The model under review builds one solid part; all positions refer to its coordinate system, in mm. Face numbers are marked on the shaded views. A direction names the side the tool comes from. Round coordinates to 2 decimals unless told otherwise and drop trailing zeros. Order: outer loops, then holes, each group sorted by start corner. A loop starts at its lowest first (then second) coordinate and runs counter-clockwise, first axis right, second up.
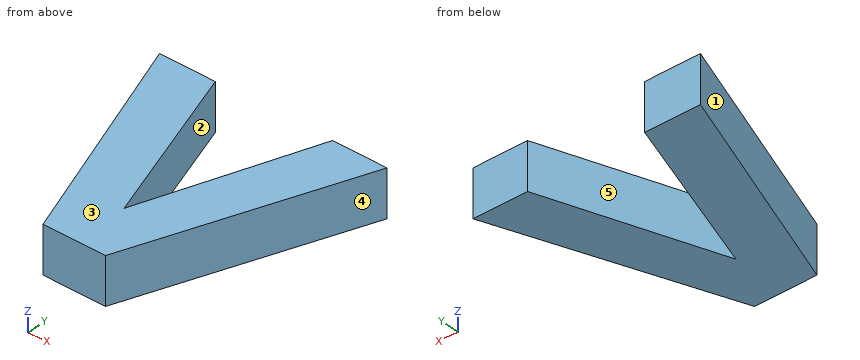
Autodesk Inventor part; units mm, degrees
ref_plane "YZ Plane" through (0, 0, 0) normal (1, 0, 0) x (0, 1, 0)
ref_plane "XZ Plane" through (0, 0, 0) normal (0, 1, 0) x (-1, 0, 0)
ref_plane "XY Plane" through (0, 0, 0) normal (0, 0, 1) x (1, 0, 0)
sketch "Sketch1" plane through (0, 0, 0) normal (0, 0, 1) x (1, 0, 0)
  line L0 (-20, -20) -> (20, -20)
  line L1 (20, -20) -> (20, 20)
  line L2 (20, 20) -> (-20, 20)
  line L3 (-20, 20) -> (-20, -20)
  line L4 (-20, 0) -> (20, 0) construction
  line L5 (0, -28) -> (0, 28) construction
  line L6 (-28, 0) -> (28, 0) construction
  point P0 (0, 0)
  dimension "d0" = 40
extrude "Extrusion1" add sketch "Sketch1" along normal blind 1.4
sketch "Sketch2" plane through (0, 0, 1.4) normal (0, 0, 1) x (1, 0, 0)
  line L0 (20, -20) -> (20, 20)
  line L1 (20, 20) -> (-20, 20)
  line L2 (-20, 20) -> (-20, -20)
  line L3 (-20, -20) -> (20, -20)
  line L4 (-17.2054, 4.9978) -> (-19.7504, 12.0011) construction
  line L5 (-19.7504, 12.0011) -> (-17.859, 11.9986) construction
  line L6 (-17.859, 11.9986) -> (-16.1741, 7.0821) construction
  line L7 (-16.1741, 7.0821) -> (-14.4762, 11.9942) construction
  line L8 (-14.4762, 11.9942) -> (-12.6247, 11.9918) construction
  line L9 (-12.6247, 11.9918) -> (-15.1882, 4.9951) construction
  line L10 (-15.1882, 4.9951) -> (-17.2054, 4.9978) construction
  line L11 (-16.1745, 6.7749) -> (-17.9305, 11.8987)
  line L12 (-17.9305, 11.8987) -> (-19.6076, 11.9009)
  line L13 (-19.6076, 11.9009) -> (-17.1353, 5.0977)
  line L14 (-17.1353, 5.0977) -> (-15.2581, 5.0952)
  line L15 (-15.2581, 5.0952) -> (-12.7678, 11.8919)
  line L16 (-12.7678, 11.8919) -> (-14.405, 11.8941)
  line L17 (-14.405, 11.8941) -> (-16.1745, 6.7749)
  point P0 (0, 0)
  dimension "d3" = 0.1
extrude "Extrusion2" cut sketch "Sketch2" against normal up to next
properties part number "V_letter"
(1) Consider section D-D (x = -17.75). Write out the cut boundary in (y, z), and give its area (3 significant figures).
Data:
outline: (6.79, 0) - (11.37, 0) - (11.37, 1.4) - (6.79, 1.4) - close
area: 6.42 mm2
(2) Consider section C-C (y = 11). Write out the cut boundary in (x, z), and give its area (3 significant figures).
Data:
outline: (-19.28, 0) - (-17.62, 0) - (-17.62, 1.4) - (-19.28, 1.4) - close; (-14.71, 0) - (-13.09, 0) - (-13.09, 1.4) - (-14.71, 1.4) - close
area: 4.59 mm2
(3) Consider section B-B (z = 0.7). Write out the cut boundary in (x, y) (1 decimal), and give its area (3 significant figures).
Data:
outline: (-19.6, 11.9) - (-17.1, 5.1) - (-15.3, 5.1) - (-12.8, 11.9) - (-14.4, 11.9) - (-16.2, 6.8) - (-17.9, 11.9) - close
area: 20.6 mm2
(4) Consider section A-A (y = 9.75). Write out the cut boundary in (x, z).
Data:
outline: (-18.83, 0) - (-17.19, 0) - (-17.19, 1.4) - (-18.83, 1.4) - close; (-15.15, 0) - (-13.55, 0) - (-13.55, 1.4) - (-15.15, 1.4) - close
(5) To check wall thickness, follow probe 1 along X at (y, z) = (8.5, 1.3); probe 2 along X at (y, z) = (9.5, 1.1); probe 3 along X at (y, z) = (5.5, 0.4). State the ranges of each line that lie inside material, in increasing order.
Data:
probe 1: x = -18.37 to -16.77, -15.58 to -14.01
probe 2: x = -18.74 to -17.11, -15.23 to -13.64
probe 3: x = -17.28 to -15.11
(6) Draft analysis for pull direction X (two halves, no side actions). For the marked faces 1, 2 and 3, state which applies: pulls with the +X half, pulls with the -X half, needs draft (parallel to the pull), parting line crosses it, or undercut.
Data:
face 1: pulls with the -X half
face 2: undercut
face 3: needs draft
(7) For the marked faces 4 and 5, list the 3-axis set-ups (+Z, -Z, +X, -X, +Y, -Y) from which the entire face can be reached by the end or side of a thin tool; tool diameter is ignored.
Data:
face 4: +Z, -Z, +X, -Y
face 5: +Z, -Z, +Y
